Source: CAD feature listing. Evaluate the final solid. Frame: model axes, mm. Face numbers are marked on the shaded views. A direction names the side the tool comes from. Coordinates: 2 decimals unless noted, no trailing zeros. One line per question, with ' | ' between items. Start each with the question number.
1. Pin query (flat end, axial travel): P1, Ø4, axis at x = 0, z = 0, coming from the +Y side; P2, Ø2, axis at y = 4.5, z = -1.5, coming from the -X side. Return the tip coordinate at first contact, or that it passes through.
2. Mould query, pull axis X, two halves, no side actions, for the marked faces 3, 4 and 5. Classes: pulls with the +X half, pulls with the -X half, needs draft (parallel to the pull), parting line crosses it, or undercut.
3. Section query A-A, the plane z = -7.25. State how many separate pieces and enclosed holes the cut face has, and give its area (3 significant figures).
4. Access query for the marked faces 1 and 2. Directions: +Z, -Z, +X, -X, +Y, -Y. A direction counts if a zero-diameter tool reaches every point of the face in a straight line with its end or side. Return the directions, or none.
5. Ray query, probe 1 along Z at (x, y) = (0, 3.5) (3 decimals); probe 2 along Y at (x, z) = (3, -0.5); probe 3 along Z at (x, y) = (-6.75, 3.5). Return the intervals inside material, ascending.
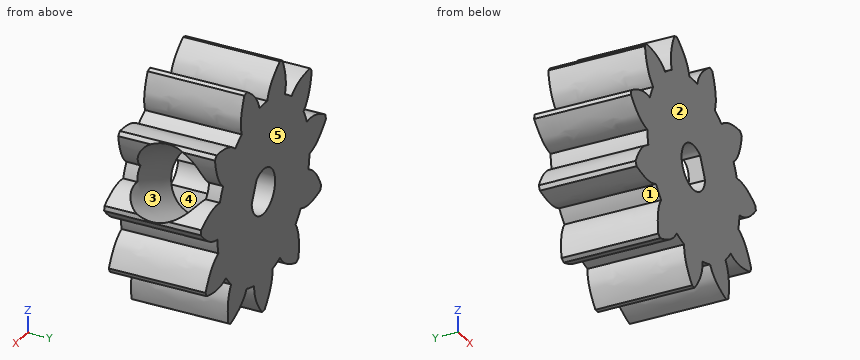
```python
from build123d import *

# Parameters (mm, degrees)
SKETCH1_R           = 6.985
BOSS_EXTRUDE1_DEPTH = 7.62
CIRPATTERN1_COUNT   = 11
CUT_EXTRUDE1_DEPTH  = 16.43236868


# Read off the part's stored shape, not the designer's step: Cut-Extrude2
with BuildPart() as part:
    # Sketch1 → Boss-Extrude1 (new body)
    with BuildSketch(Plane(origin=(0, 0, 0), x_dir=(1, 0, 0), z_dir=(0, 1, 0))):
        Circle(SKETCH1_R)
        with BuildLine():
            add(Edge.make_bspline(
                [(1.387604422, 6.84578549), (1.423643939, 7.597190899), (0.984603354, 8.544581789), (0.361474483, 9.332383529), (0.192044664, 9.523063785)],
                knots=[0, 0, 0, 0, 0.250134969, 0.335748037, 0.335748037, 0.335748037, 0.335748037], degree=3))
            ThreePointArc((0.192044664, 9.523063785), (0, 9.525), (-0.192044664, 9.523063785))
            add(Edge.make_bspline(
                [(-1.387604422, 6.84578549), (-1.423643939, 7.597190899), (-0.984603354, 8.544581789), (-0.361474483, 9.332383529), (-0.192044664, 9.523063785)],
                knots=[0, 0, 0, 0, 0.250134969, 0.335748037, 0.335748037, 0.335748037, 0.335748037], degree=3))
            ThreePointArc((-1.387604422, 6.84578549), (0, 6.985), (1.387604422, 6.84578549))
        make_face()
    boss_extrude1 = extrude(amount=BOSS_EXTRUDE1_DEPTH)

    # CirPattern1: Boss-Extrude1 ×11 about axis
    cirpattern1_axis = Axis((0, 7.62, 0), (0, -1, 0))
    for i in range(1, CIRPATTERN1_COUNT):
        add(boss_extrude1.rotate(cirpattern1_axis, i * 360 / CIRPATTERN1_COUNT))

    # Sketch2 → Cut-Extrude1 (cut, through all)
    with BuildSketch(Plane(origin=(0, 7.62, 0), x_dir=(1, 0, 0), z_dir=(0, 1, 0))):
        with BuildLine():
            Line((1.769949078, 0.169009645), (1.031341185, -1.448316043))
            ThreePointArc((1.031341185, -1.448316043), (-1.617325688, 0.738607893), (1.769949078, 0.169009645))
        make_face()
    extrude(amount=-CUT_EXTRUDE1_DEPTH, mode=Mode.SUBTRACT)

    # Cut-Extrude2 outline → Cut-Extrude2 (revolve, cut)
    with BuildSketch(Plane(origin=(0, 3.81, 0), x_dir=(0, 1, 0), z_dir=(0.41541501300188993, 0, -0.9096319953545169))):
        Polygon((0, 1.539793168), (2.667, 1.539793168), (2.800559609, 9.191418023), (0, 9.191418023), align=None)
    revolve(axis=Axis((0, 3.81, 0), (0.9096319953545169, 0, 0.41541501300188993)), mode=Mode.SUBTRACT)


solid = part.part
```
Taken from the geometry:
1) P1: y = 7.62 | P2: x = -7.98
2) face 3: undercut | face 4: undercut | face 5: needs draft
3) separate pieces: 3 | enclosed holes: 0 | area: 54.4 mm^2
4) face 1: +Y, -Y | face 2: +Z, -Z, +X, -X, -Y
5) probe 1: -9.525 to -1.778, 1.778 to 6.985 | probe 2: 0 to 1.73, 5.89 to 7.62 | probe 3: -4.39 to 2.37, 4.23 to 6.38
